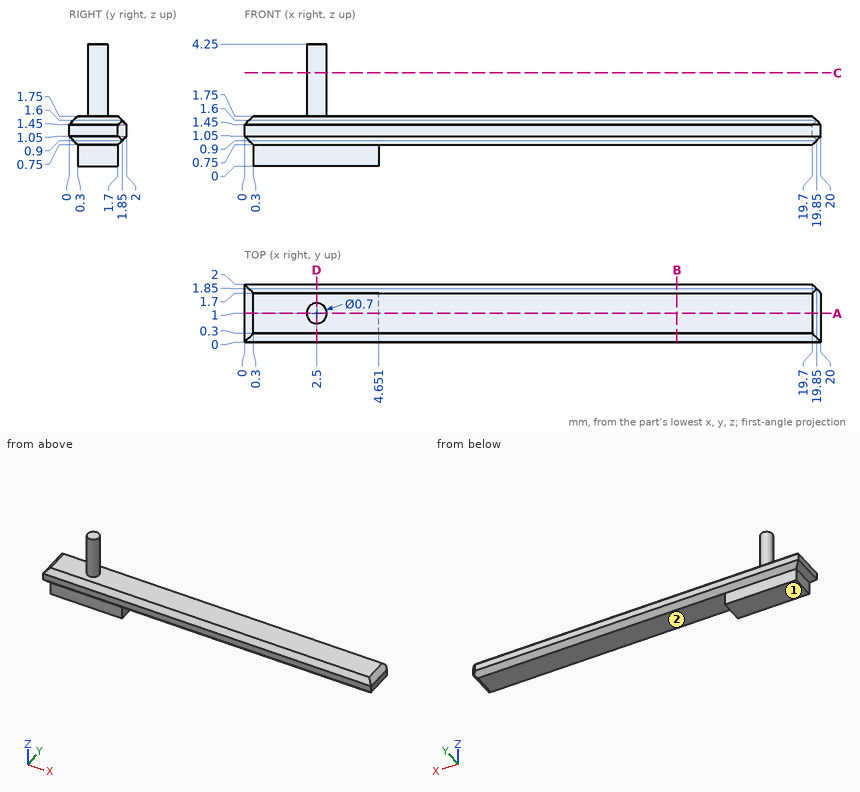
Drawing for the job (mm, zero at the part's lowest x, y, z). A direction names the side the tool comes from. Round coordinates to 2 decimals unless told otherwise and drop trailing zeros. Order: outer loops, then holes, each group sorted by start corner. A loop starts at its lowest first (then second) coordinate and runs counter-clockwise, first axis right, second up. Notation, with made-up numbers: M 65,75 L 93,75 A18 cw 93,85 Z; hole C -34,32 d11. An arc over 180 degrees is marked long. Use one line per item in the form item = value.
Q1. Saw through at D-D on x = 2.5. Give the cut face in (y, z).
Recorded:
outline = M 0,1.05 L 0.3,0.75 L 0.3,0 L 1.7,0 L 1.7,0.75 L 2,1.05 L 2,1.45 L 1.7,1.75 L 1.35,1.75 L 1.35,4.25 L 0.65,4.25 L 0.65,1.75 L 0.3,1.75 L 0,1.45 Z
Q2. Which spindle directions (+Z, -Z, +X, -X, +Y, -Y) get a long thin tool onto all of the face, cutting with end or side? Do the marked faces 1 and 2. Say none if no direction does.
Recorded:
face_1 = -Z, +X, -X, +Y, -Y
face_2 = -Z, +X, +Y, -Y
Q3. Saw through at A-A on y = 1. Give the cut face in (x, z).
Recorded:
outline = M 0,1.05 L 0.3,0.75 L 0.3,0 L 4.65,0 L 4.65,0.75 L 19.7,0.75 L 20,1.05 L 20,1.45 L 19.7,1.75 L 2.85,1.75 L 2.85,4.25 L 2.15,4.25 L 2.15,1.75 L 0.3,1.75 L 0,1.45 Z
Q4. Saw through at C-C on z = 3.25. Give the cut face in (x, y).
Recorded:
outline = C 2.5,1 d0.7
Q5. Saw through at B-B on x = 15. Give the cut face in (y, z).
Recorded:
outline = M 0,1.05 L 0.3,0.75 L 1.7,0.75 L 2,1.05 L 2,1.45 L 1.7,1.75 L 0.3,1.75 L 0,1.45 Z
Q6. Flat gauge pins, fed straight in: P1, Ø0.8, axis at y = 1, z = 0.5, coming from the -X side; P2, Ø1.1, axis at x = 9, y = 1, coming from the +Z side; P3, Ø1.1, axis at x = 13.5, y = 1, coming from the -Z side. Where does each tip first touch, or does it go through?
Recorded:
P1 = 0.15
P2 = 1.75
P3 = 0.75
Q7. Probe L1, parallel to Y at x = 2.5, z = 0.4; L2, parallel to Z at x = 10.5, y = 0.65; L3, parallel to Z at x = 2, y = 0.85. List the from-to ranges inside material, lowest first.
Recorded:
L1 = 0.3 to 1.7
L2 = 0.75 to 1.75
L3 = 0 to 1.75
